```python
from build123d import *

# Parameters (mm, degrees)
SKETCH_1_W           = 300
SKETCH_1_H           = 100
EXTRUDE_1_DEPTH      = 16
SKETCH_2_W           = 30
SKETCH_2_H           = 30
CUT_EXTRUDE_1_DEPTH  = 8
SKETCH_3_R           = 12.5
CUT_EXTRUDE_2_DEPTH  = 14
CUT_EXTRUDE_3_REACH  = 318.632
SKETCH_4_W           = 50
SKETCH_4_H           = 35
SKETCH_7_W           = 35
SKETCH_7_H           = 16
EXTRUDE_2_DEPTH      = 20
SKETCH_8_W           = 35
SKETCH_8_H           = 16
EXTRUDE_3_DEPTH      = 20
SKETCH_9_W           = 20
SKETCH_9_H           = 10
EXTRUDE_4_DEPTH      = 25
FILLET_1_R           = 1
FILLET_2_R           = 1
SKETCH_13_W          = 35
SKETCH_13_H          = 16
EXTRUDE_6_DEPTH      = 4
SKETCH_14_W          = 35
SKETCH_14_H          = 16
EXTRUDE_7_DEPTH      = 4
SKETCH_17_W          = 35
SKETCH_17_H          = 16
EXTRUDE_8_DEPTH      = 1
SKETCH_18_W          = 35
SKETCH_18_H          = 16
EXTRUDE_9_DEPTH      = 1
SKETCH_19_R          = 2.25
CUT_EXTRUDE_8_DEPTH  = 5
CUT_EXTRUDE_START    = -7
SKETCH_20_R          = 2.25
CUT_EXTRUDE_9_DEPTH  = 7
CUT_EXTRUDE_15_DEPTH = 2
SKETCH_28_R          = 2.25
CUT_EXTRUDE_18_DEPTH = 5
SKETCH_30_R          = 1.5
CUT_EXTRUDE_20_DEPTH = 4


with BuildPart() as part:
    # 草图1 → 凸台-拉伸1 (new body)
    with BuildSketch(Plane(origin=(0, 0, 0), x_dir=(1, 0, 0), z_dir=(0, 1, 0))):
        with Locations((-150, 50)):
            Rectangle(SKETCH_1_W, SKETCH_1_H)
    extrude(amount=EXTRUDE_1_DEPTH)

    # 草图2 → 切除-拉伸1 (cut)
    with BuildSketch(Plane(origin=(0, 16, 0), x_dir=(1, 0, 0), z_dir=(0, 1, 0))):
        with Locations((-150, 50)):
            Rectangle(SKETCH_2_W, SKETCH_2_H)
    extrude(amount=-CUT_EXTRUDE_1_DEPTH, mode=Mode.SUBTRACT)

    # 草图3 → 切除-拉伸2 (cut)
    with BuildSketch(Plane(origin=(0, 8, 0), x_dir=(1, 0, 0), z_dir=(0, 1, 0))):
        with Locations(Location((-150, 50, 0), (0, 0, 270))):
            Circle(SKETCH_3_R)
    extrude(amount=-CUT_EXTRUDE_2_DEPTH, mode=Mode.SUBTRACT)

    # 草图4 → 切除-拉伸3 (cut, up to next)
    with BuildSketch(Plane(origin=(0, 16, 0), x_dir=(1, 0, 0), z_dir=(0, 1, 0)), mode=Mode.PRIVATE) as cut_extrude_3_sk1:
        with Locations((-270, 72.5)):
            Rectangle(SKETCH_4_W, SKETCH_4_H)
    cut_extrude_3_tool1 = extrude(cut_extrude_3_sk1.sketch, amount=-CUT_EXTRUDE_3_REACH, mode=Mode.PRIVATE) & part.part
    # 草图4 → 切除-拉伸3 (cut, up to next)
    with BuildSketch(Plane(origin=(0, 16, 0), x_dir=(1, 0, 0), z_dir=(0, 1, 0)), mode=Mode.PRIVATE) as cut_extrude_3_sk2:
        with Locations((-270, 27.5)):
            Rectangle(SKETCH_4_W, SKETCH_4_H)
    cut_extrude_3_tool2 = extrude(cut_extrude_3_sk2.sketch, amount=-CUT_EXTRUDE_3_REACH, mode=Mode.PRIVATE) & part.part
    # 草图4 → 切除-拉伸3 (cut, up to next)
    with BuildSketch(Plane(origin=(0, 16, 0), x_dir=(1, 0, 0), z_dir=(0, 1, 0)), mode=Mode.PRIVATE) as cut_extrude_3_sk3:
        with Locations((-210, 72.5)):
            Rectangle(SKETCH_4_W, SKETCH_4_H)
    cut_extrude_3_tool3 = extrude(cut_extrude_3_sk3.sketch, amount=-CUT_EXTRUDE_3_REACH, mode=Mode.PRIVATE) & part.part
    # 草图4 → 切除-拉伸3 (cut, up to next)
    with BuildSketch(Plane(origin=(0, 16, 0), x_dir=(1, 0, 0), z_dir=(0, 1, 0)), mode=Mode.PRIVATE) as cut_extrude_3_sk4:
        with Locations((-210, 27.5)):
            Rectangle(SKETCH_4_W, SKETCH_4_H)
    cut_extrude_3_tool4 = extrude(cut_extrude_3_sk4.sketch, amount=-CUT_EXTRUDE_3_REACH, mode=Mode.PRIVATE) & part.part
    # 草图4 → 切除-拉伸3 (cut, up to next)
    with BuildSketch(Plane(origin=(0, 16, 0), x_dir=(1, 0, 0), z_dir=(0, 1, 0)), mode=Mode.PRIVATE) as cut_extrude_3_sk5:
        with Locations((-30, 27.5)):
            Rectangle(SKETCH_4_W, SKETCH_4_H)
    cut_extrude_3_tool5 = extrude(cut_extrude_3_sk5.sketch, amount=-CUT_EXTRUDE_3_REACH, mode=Mode.PRIVATE) & part.part
    # 草图4 → 切除-拉伸3 (cut, up to next)
    with BuildSketch(Plane(origin=(0, 16, 0), x_dir=(1, 0, 0), z_dir=(0, 1, 0)), mode=Mode.PRIVATE) as cut_extrude_3_sk6:
        with Locations((-90, 27.5)):
            Rectangle(SKETCH_4_W, SKETCH_4_H)
    cut_extrude_3_tool6 = extrude(cut_extrude_3_sk6.sketch, amount=-CUT_EXTRUDE_3_REACH, mode=Mode.PRIVATE) & part.part
    # 草图4 → 切除-拉伸3 (cut, up to next)
    with BuildSketch(Plane(origin=(0, 16, 0), x_dir=(1, 0, 0), z_dir=(0, 1, 0)), mode=Mode.PRIVATE) as cut_extrude_3_sk7:
        with Locations((-90, 72.5)):
            Rectangle(SKETCH_4_W, SKETCH_4_H)
    cut_extrude_3_tool7 = extrude(cut_extrude_3_sk7.sketch, amount=-CUT_EXTRUDE_3_REACH, mode=Mode.PRIVATE) & part.part
    # 草图4 → 切除-拉伸3 (cut, up to next)
    with BuildSketch(Plane(origin=(0, 16, 0), x_dir=(1, 0, 0), z_dir=(0, 1, 0)), mode=Mode.PRIVATE) as cut_extrude_3_sk8:
        with Locations((-30, 72.5)):
            Rectangle(SKETCH_4_W, SKETCH_4_H)
    cut_extrude_3_tool8 = extrude(cut_extrude_3_sk8.sketch, amount=-CUT_EXTRUDE_3_REACH, mode=Mode.PRIVATE) & part.part
    add(cut_extrude_3_tool1.solids().sort_by_distance((-270, 16, -72.5))[0], mode=Mode.SUBTRACT)
    add(cut_extrude_3_tool2.solids().sort_by_distance((-270, 16, -27.5))[0], mode=Mode.SUBTRACT)
    add(cut_extrude_3_tool3.solids().sort_by_distance((-210, 16, -72.5))[0], mode=Mode.SUBTRACT)
    add(cut_extrude_3_tool4.solids().sort_by_distance((-210, 16, -27.5))[0], mode=Mode.SUBTRACT)
    add(cut_extrude_3_tool5.solids().sort_by_distance((-30, 16, -27.5))[0], mode=Mode.SUBTRACT)
    add(cut_extrude_3_tool6.solids().sort_by_distance((-90, 16, -27.5))[0], mode=Mode.SUBTRACT)
    add(cut_extrude_3_tool7.solids().sort_by_distance((-90, 16, -72.5))[0], mode=Mode.SUBTRACT)
    add(cut_extrude_3_tool8.solids().sort_by_distance((-30, 16, -72.5))[0], mode=Mode.SUBTRACT)

    # 草图7 → 凸台-拉伸2 (add)
    with BuildSketch(Plane.ZY.offset(185)):
        with Locations((-27.5, 8)):
            Rectangle(SKETCH_7_W, SKETCH_7_H)
        with Locations((-72.5, 8)):
            Rectangle(SKETCH_7_W, SKETCH_7_H)
    extrude(amount=EXTRUDE_2_DEPTH)

    # 草图8 → 凸台-拉伸3 (add)
    with BuildSketch(Plane(origin=(-115, 0, 0), x_dir=(0, 0, -1), z_dir=(1, 0, 0))):
        with Locations((27.5, 8)):
            Rectangle(SKETCH_8_W, SKETCH_8_H)
        with Locations((72.5, 8)):
            Rectangle(SKETCH_8_W, SKETCH_8_H)
    extrude(amount=EXTRUDE_3_DEPTH)

    # 草图9 → 凸台-拉伸4 (add)
    with BuildSketch(Plane.XZ):
        with Locations((-250, -95)):
            Rectangle(SKETCH_9_W, SKETCH_9_H)
    extrude(amount=EXTRUDE_4_DEPTH)

    # 圆角1
    fillet_1_edges = [part.edges().sort_by_distance(p)[0] for p in [
        (-150, 8, -62.5),
    ]]
    fillet(fillet_1_edges, radius=FILLET_1_R)

    # 圆角2
    fillet_2_edges = [part.edges().sort_by_distance(p)[0] for p in [
        (-135, 16, -50),
        (-150, 16, -65),
        (-165, 16, -50),
        (-150, 16, -35),
    ]]
    fillet(fillet_2_edges, radius=FILLET_2_R)

    # 草图13 → 凸台-拉伸6 (add)
    with BuildSketch(Plane.ZY.offset(5)):
        with Locations((-72.5, 8)):
            Rectangle(SKETCH_13_W, SKETCH_13_H)
        with Locations((-27.5, 8)):
            Rectangle(SKETCH_13_W, SKETCH_13_H)
    extrude(amount=EXTRUDE_6_DEPTH)

    # 草图14 → 凸台-拉伸7 (add)
    with BuildSketch(Plane(origin=(-295, 0, 0), x_dir=(0, 0, -1), z_dir=(1, 0, 0))):
        with Locations((72.5, 8)):
            Rectangle(SKETCH_14_W, SKETCH_14_H)
        with Locations((27.5, 8)):
            Rectangle(SKETCH_14_W, SKETCH_14_H)
    extrude(amount=EXTRUDE_7_DEPTH)

    # 草图17 → 凸台-拉伸8 (add)
    with BuildSketch(Plane(origin=(-291, 0, 0), x_dir=(0, 0, -1), z_dir=(1, 0, 0))):
        with Locations((27.5, 8)):
            Rectangle(SKETCH_17_W, SKETCH_17_H)
        with Locations((72.5, 8)):
            Rectangle(SKETCH_17_W, SKETCH_17_H)
    extrude(amount=EXTRUDE_8_DEPTH)

    # 草图18 → 凸台-拉伸9 (add)
    with BuildSketch(Plane.ZY.offset(9)):
        with Locations((-27.5, 8)):
            Rectangle(SKETCH_18_W, SKETCH_18_H)
        with Locations((-72.5, 8)):
            Rectangle(SKETCH_18_W, SKETCH_18_H)
    extrude(amount=EXTRUDE_9_DEPTH)

    # 草图19 → 切除-拉伸8 (cut)
    with BuildSketch(Plane(origin=(0, 16, 0), x_dir=(1, 0, 0), z_dir=(0, 1, 0))):
        with Locations(Location((-295, 95, 0), (0, 0, 270))):
            Circle(SKETCH_19_R)
        with Locations(Location((-295, 5, 0), (0, 0, 90))):
            Circle(SKETCH_19_R)
        with Locations(Location((-5, 5, 0), (0, 0, 270))):
            Circle(SKETCH_19_R)
        with Locations(Location((-5, 95, 0), (0, 0, 90))):
            Circle(SKETCH_19_R)
    extrude(amount=-CUT_EXTRUDE_8_DEPTH, mode=Mode.SUBTRACT)

    # 草图20 → 切除-拉伸9 (cut)
    with BuildSketch(Plane.XZ.offset(CUT_EXTRUDE_START)):
        with Locations(Location((-295, -95, 0), (0, 0, 90))):
            Circle(SKETCH_20_R)
        with Locations(Location((-295, -5, 0), (0, 0, 270))):
            Circle(SKETCH_20_R)
        with Locations(Location((-5, -95, 0), (0, 0, 270))):
            Circle(SKETCH_20_R)
        with Locations(Location((-5, -5, 0), (0, 0, 90))):
            Circle(SKETCH_20_R)
    extrude(amount=CUT_EXTRUDE_9_DEPTH, mode=Mode.SUBTRACT)

    # 草图26 → 切除-拉伸15 (cut)
    with BuildSketch(Plane.XZ):
        Polygon((-260, -90), (-290, -90), (-290, -55), (-245, -55), (-245, -90), (-240, -90), (-240, -100), (0, -100), (0, 0), (-300, 0), (-300, -100), (-260, -100), align=None)
    extrude(amount=-CUT_EXTRUDE_15_DEPTH, mode=Mode.SUBTRACT)

    # 草图28 → 切除-拉伸18 (cut)
    with BuildSketch(Plane(origin=(0, 16, 0), x_dir=(1, 0, 0), z_dir=(0, 1, 0))):
        with Locations(Location((-105.002761288, 55.000000147, 0), (0, 0, 270))):
            Circle(SKETCH_28_R)
        with Locations(Location((-105, 81, 0), (0, 0, 270))):
            Circle(SKETCH_28_R)
        with Locations(Location((-120, 78.499971194, 0), (0, 0, 270))):
            Circle(SKETCH_28_R)
        with Locations(Location((-120, 95.5, 0), (0, 0, 270))):
            Circle(SKETCH_28_R)
        with Locations(Location((-167.000079641, 78.5, 0), (0, 0, 270))):
            Circle(SKETCH_28_R)
        with Locations(Location((-167.000079641, 95.5, 0), (0, 0, 270))):
            Circle(SKETCH_28_R)
        with Locations(Location((-195, 54.99995086, 0), (0, 0, 270))):
            Circle(SKETCH_28_R)
        with Locations(Location((-195, 81, 0), (0, 0, 270))):
            Circle(SKETCH_28_R)
    extrude(amount=-CUT_EXTRUDE_18_DEPTH, mode=Mode.SUBTRACT)

    # 草图30 → 切除-拉伸20 (cut)
    with BuildSketch(Plane(origin=(0, 11, 0), x_dir=(1, 0, 0), z_dir=(0, 1, 0))):
        with Locations(Location((-195, 81, 0), (0, 0, 270))):
            Circle(SKETCH_30_R)
        with Locations(Location((-195, 54.99995086, 0), (0, 0, 270))):
            Circle(SKETCH_30_R)
        with Locations(Location((-167.000079641, 95.5, 0), (0, 0, 270))):
            Circle(SKETCH_30_R)
        with Locations(Location((-167.000079641, 78.5, 0), (0, 0, 270))):
            Circle(SKETCH_30_R)
        with Locations(Location((-120, 95.5, 0), (0, 0, 270))):
            Circle(SKETCH_30_R)
        with Locations(Location((-120, 78.499971194, 0), (0, 0, 270))):
            Circle(SKETCH_30_R)
        with Locations(Location((-105, 81, 0), (0, 0, 270))):
            Circle(SKETCH_30_R)
        with Locations(Location((-105.002761288, 55.000000147, 0), (0, 0, 270))):
            Circle(SKETCH_30_R)
    extrude(amount=-CUT_EXTRUDE_20_DEPTH, mode=Mode.SUBTRACT)


solid = part.part
```
Can you work these out from the model? Positions are in its coordinate system, mm. A direction names the side the tool comes from. Coordinates: 2 decimals unless noted, no trailing zeros. Write each loop counter-clockwise with the first axis right and the second up, starting at its lowest first coordinate (ties: lowest second). Pieces come first, ordered by that corner, then holes. Notation, with made-up numbers: (66, 36.5) - (124, 36.5) arc R21 ccw to (124, 47.5) - close; hole circle Ø4 at (77.25, 50.5). An arc over 180 degrees is marked (long way). Return JSON: item names as keys, results as strings.
Q1. I'm going to push flat-ended pins straight in: pin 1 Ø10 at (x, z) = (-128, -23) entering from -Y; pin 2 Ø3.5 at (x, z) = (-5, -95) entering from -Y; pin 3 Ø1.3 at (x, z) = (-294.5, -94.5) entering from +Y. Where does each tip first touch, or does it pass through?
Computed values:
{"pin 1": "stops at y = 2", "pin 2": "stops at y = 7", "pin 3": "stops at y = 11"}
Q2. Please list where these lines run through material, in increasing order: L1, parallel to X at y = 7, z = -85.5; L2, parallel to X at y = 7.8, z = -95.5; L3, parallel to Z at x = -218, y = 14. Write a range as from..to.
Computed values:
{"L1": "x = -300..-290, -245..-235, -205..-95, -65..-55, -10..0", "L2": "x = -300..-168.5, -165.5..-121.5, -118.5..0", "L3": "z = -100..-90, -55..-45, -10..0"}
Q3. On a 3-axis mill with a long thin cutter (end or side, diameter ignored), from which of +Z, -Z, +X, -X, +Y, -Y can I reach the whole of each face in a straight line? I mean faces 5 (the flat face through (-165, 12, -50)), 6 (the flat face through (-220, 9, -55)), 7 (the flat face through (0, 9, -49)). Say none if no direction works.
Computed values:
{"face 5": "+Y", "face 6": "+Y, -Y", "face 7": "+Z, -Z, +X, +Y, -Y"}
Q4. If we section it at A-A (x = -70): Please give me the cut outline in (y, z).
Computed values:
{"outline": "(2, -100) - (16, -100) - (16, -90) - (2, -90) - close; (2, -55) - (16, -55) - (16, -45) - (2, -45) - close; (2, -10) - (16, -10) - (16, 0) - (2, 0) - close"}
Q5. Thinking about a two-plate mould opening in X: for faces 1 (the flat face through (-300, 9, -49)), 2 (the flat face through (-152, 2, -27)), 3 (the flat face through (-240, -12, -95)), 4 (the flat face through (-235, 9, -72)), which applies, +X half, -X half, draft (parallel to the pull), parting line (faces both ways), or undercut?
Computed values:
{"face 1": "-X half", "face 2": "draft", "face 3": "+X half", "face 4": "undercut"}
Q6. If we section it at B-B (z = -50): Please give me the cut outline in (x, y), then the cut area to 3 significant figures.
Computed values:
{"outline": "(-300, 2) - (-162.5, 2) - (-162.5, 7) arc R1 ccw to (-163.5, 8) - (-165, 8) - (-165, 15) arc R1 ccw to (-166, 16) - (-300, 16) - close; (-137.5, 2) - (0, 2) - (0, 16) - (-134, 16) arc R1 ccw to (-135, 15) - (-135, 8) - (-136.5, 8) arc R1 ccw to (-137.5, 7) - close", "area": "3,810 mm2"}
Q7. If we section it at D-D (x = -249.5): Please give me the cut outline in (y, z).
Computed values:
{"outline": "(-25, -100) - (16, -100) - (16, -90) - (-25, -90) - close; (2, -55) - (16, -55) - (16, -45) - (2, -45) - close; (2, -10) - (16, -10) - (16, 0) - (2, 0) - close"}
Q8. If we section it at C-C (z = -15): Please give me the cut outline in (x, y), then the cut area to 3 significant figures.
Computed values:
{"outline": "(-300, 2) - (-290, 2) - (-290, 16) - (-300, 16) - close; (-245, 2) - (-235, 2) - (-235, 16) - (-245, 16) - close; (-205, 2) - (-95, 2) - (-95, 16) - (-205, 16) - close; (-65, 2) - (-55, 2) - (-55, 16) - (-65, 16) - close; (-10, 2) - (0, 2) - (0, 16) - (-10, 16) - close", "area": "2,100 mm2"}
